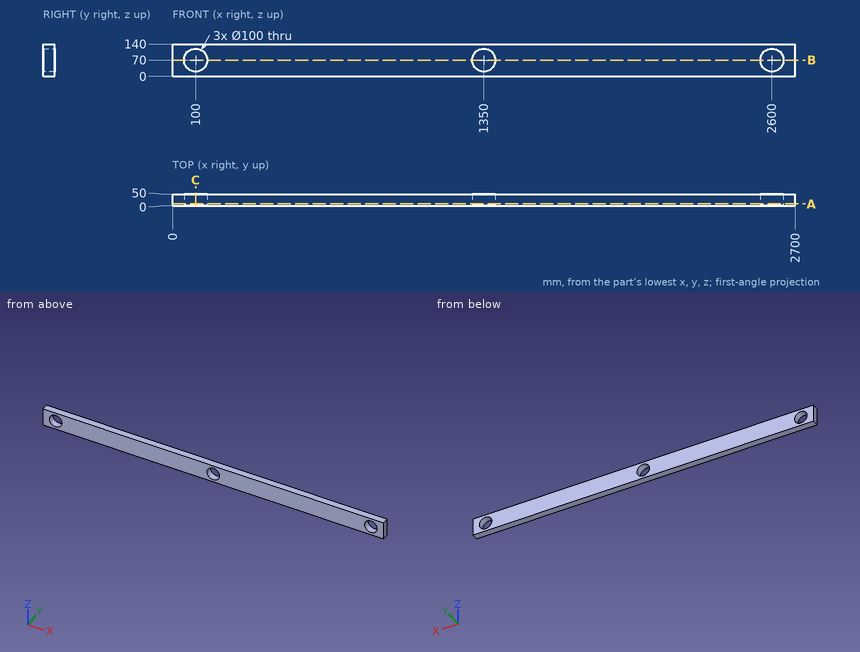
The figure shows three views and two pictorial views of one solid part (mm, origin at its lowest corner). Answer the questions. Round coordinates to 2 decimals unless told otherwise and drop trailing zeros. Loops run counter-clockwise (first coordinate to the right, second up) from the corner with the lowest first, then second, coordinate; pieces in that order, holes last. Notation, with made-up numbers: M 5,46.25 L 57,46.25 A18 ccw 57,73.25 Z; hole C 52.25,-9 d9. An arc over 180 degrees is marked long. Return JSON: item names as keys, results as strings.
Q1. Find section C-C, the plane x = 100. Determine the outline of the cut face in (y, z).
Results list:
{"outline": "M 0,0 L 50,0 L 50,20 L 0,20 Z; M 0,120 L 50,120 L 50,140 L 0,140 Z"}
Q2. Find the intervals of material crossed by line 1 along X through (y, z) = (34.5, 65); line 2 along X through (y, z) = (40, 67); line 3 along Z through (x, y) = (2600, 17), in increasing order. Write a range as from..to.
Results list:
{"line 1": "x = 0..50.25, 149.75..1300.25, 1399.75..2550.25, 2649.75..2700", "line 2": "x = 0..50.09, 149.91..1300.09, 1399.91..2550.09, 2649.91..2700", "line 3": "z = 0..20, 120..140"}
Q3. Find section B-B, the plane z = 70. Determine the outline of the cut face in (x, y), plus the area to 3 significant figures.
Results list:
{"outline": "M 0,0 L 50,0 L 50,50 L 0,50 Z; M 150,0 L 1300,0 L 1300,50 L 150,50 Z; M 1400,0 L 2550,0 L 2550,50 L 1400,50 Z; M 2650,0 L 2700,0 L 2700,50 L 2650,50 Z", "area": "120,000 mm2"}
Q4. Find section A-A, the plane y = 8.5. Determine the outline of the cut face in (x, z).
Results list:
{"outline": "M 0,0 L 2700,0 L 2700,140 L 0,140 Z; hole C 100,70 d100; hole C 1350,70 d100; hole C 2600,70 d100"}
